Geometry check sheet. Reference: the model listing, model coordinates, mm. A direction names the side the tool comes from. Give positions to 0.01 mm unless a question says otherwise; leave off trailing zeros. Order: outer loops, then holes, each group sorted by start corner. A loop starts at its lowest first (then second) coordinate and runs counter-clockwise, first axis right, second up.
from build123d import *

# Parameters (mm, degrees)
SKETCH2_W           = 50
SKETCH2_H           = 170
BOSS_EXTRUDE1_DEPTH = 50
SKETCH3_W           = 44
SKETCH3_H           = 164
CUT_EXTRUDE1_DEPTH  = 47
FILLET2_R           = 2
SKETCH4_W           = 2
SKETCH4_H           = 166
BOSS_EXTRUDE2_DEPTH = 2
CUT_EXTRUDE2_DEPTH  = 170
CUT_EXTRUDE5_DEPTH  = 10


with BuildPart() as part:
    # Sketch2 → Boss-Extrude1 (new body)
    with BuildSketch(Plane.XY):
        Rectangle(SKETCH2_W, SKETCH2_H)
    extrude(amount=BOSS_EXTRUDE1_DEPTH)

    # Sketch3 → Cut-Extrude1 (cut)
    with BuildSketch(Plane.XY.offset(50)):
        Rectangle(SKETCH3_W, SKETCH3_H)
    extrude(amount=-CUT_EXTRUDE1_DEPTH, mode=Mode.SUBTRACT)

    # Fillet2
    fillet2_edges = [part.edges().sort_by_distance(p)[0] for p in [
        (0, 85, 0),
        (25, 0, 0),
        (0, -85, 0),
        (-25, 0, 0),
        (-25, 85, 25),
        (25, 85, 25),
        (25, -85, 25),
        (-25, -85, 25),
    ]]
    fillet(fillet2_edges, radius=FILLET2_R)

    # Sketch4 → Boss-Extrude2 (add)
    with BuildSketch(Plane(origin=(25, 0, 0), x_dir=(0, 0, -1), z_dir=(1, 0, 0))):
        with Locations((-49, 0)):
            Rectangle(SKETCH4_W, SKETCH4_H)
    extrude(amount=BOSS_EXTRUDE2_DEPTH)

    # Sketch5 → Cut-Extrude2 (cut)
    with BuildSketch(Plane.XZ.offset(83)):
        Polygon((25, 48), (27, 50), (27, 48), align=None)
    extrude(amount=-CUT_EXTRUDE2_DEPTH, mode=Mode.SUBTRACT)

    # Sketch9 → Cut-Extrude5 (cut)
    with BuildSketch(Plane(origin=(0, 85, 0), x_dir=(1, 0, 0), z_dir=(0, 1, 0))):
        with BuildLine():
            Line((3.750279021, -16.895768884), (3.750279021, -50))
            ThreePointArc((3.750279021, -50), (0, -53.750279021), (-3.750279021, -50))
            Line((-3.750279021, -50), (-3.750279021, -16.895768884))
            ThreePointArc((-3.750279021, -16.895768884), (0, -13.145489863), (3.750279021, -16.895768884))
        make_face()
    extrude(amount=-CUT_EXTRUDE5_DEPTH, mode=Mode.SUBTRACT)


solid = part.part
Item 1: Sectioned sample at A-A (x = -8). Enter the section's corners in (y, z), and give its area (3 significant figures).
Reported:
outline: (-85, 2) arc R2 ccw to (-83, 0) - (83, 0) arc R2 ccw to (85, 2) - (85, 50) - (82, 50) - (82, 3) - (-82, 3) - (-82, 50) - (-85, 50) - close
area: 790 mm2
Item 2: Sectioned sample at B-B (z = 41). Enter the section's corners in (x, y).
Reported:
outline: (-25, -83) arc R2 ccw to (-23, -85) - (23, -85) arc R2 ccw to (25, -83) - (25, 83) arc R2 ccw to (23, 85) - (3.75, 85) - (3.75, 82) - (22, 82) - (22, -82) - (-22, -82) - (-22, 82) - (-3.75, 82) - (-3.75, 85) - (-23, 85) arc R2 ccw to (-25, 83) - close
Item 3: Sectioned sample at D-D (x = 0). Enter the section's corners in (y, z).
Reported:
outline: (-85, 2) arc R2 ccw to (-83, 0) - (83, 0) arc R2 ccw to (85, 2) - (85, 13.15) - (82, 13.15) - (82, 3) - (-82, 3) - (-82, 50) - (-85, 50) - close
Item 4: Scan lines: L1, parallel to Y at x = -14, z = 7; L2, parallel to X at y = 78.5, z = 22; L3, parallel to Z at x = 12.5, y = 66.5. Record each from-to range of solid material in increasing order.
Reported:
L1: y = -85 to -82, 82 to 85
L2: x = -25 to -22, 22 to 25
L3: z = 0 to 3
Item 5: Gauge pin test, flat ends, axial feed: pin 1 (1 mm diameter, centred on y = 9, z = 23, fed in from +X); pin 2 (1.6 mm diameter, centred on x = 26.5, z = 49, fed in from +Y); pin 3 (4 mm diameter, centred on x = -4, y = 17.5, fed in from +Z). Record the tip position at first contact, or that the pin passes through.
Reported:
pin 1: stops at x = 25
pin 2: stops at y = 83
pin 3: stops at z = 3
Item 6: Set-up check for faces 4 (the flat face through (0, 1, 3)), 5 (the flat face through (24, -13, 50)), 6 (the flat face through (25, -1, 25)), 7 (the flat face through (-3.75, 84, 34)), 8 (the flat face through (-5, 85, 26)): record each of +Z, -Z, +X, -X, +Y, -Y from which the full face is reachable in a straight line by a thin tool's end or side.
Reported:
face 4: +Z
face 5: +Z, +X, -X, +Y, -Y
face 6: -Z, +X, +Y, -Y
face 7: +Z, +Y
face 8: +Z, -Z, +X, -X, +Y
Item 7: Draft check along X on faces 1 (the flat face through (0, -85, 26)), 2 (the flat face through (22, -1, 27)), 3 (the flat face through (-25, -1, 26)). Enter one of: released by +X, released by -X, zero draft, split by the parting line, or undercut.
Reported:
face 1: zero draft
face 2: undercut
face 3: released by -X
Item 8: Sectioned sample at C-C (y = -46.5). Enter the section's corners in (x, z), and give its area (3 significant figures).
Reported:
outline: (-25, 2) arc R2 ccw to (-23, 0) - (23, 0) arc R2 ccw to (25, 2) - (25, 48) - (27, 50) - (22, 50) - (22, 3) - (-22, 3) - (-22, 50) - (-25, 50) - close
area: 432 mm2
